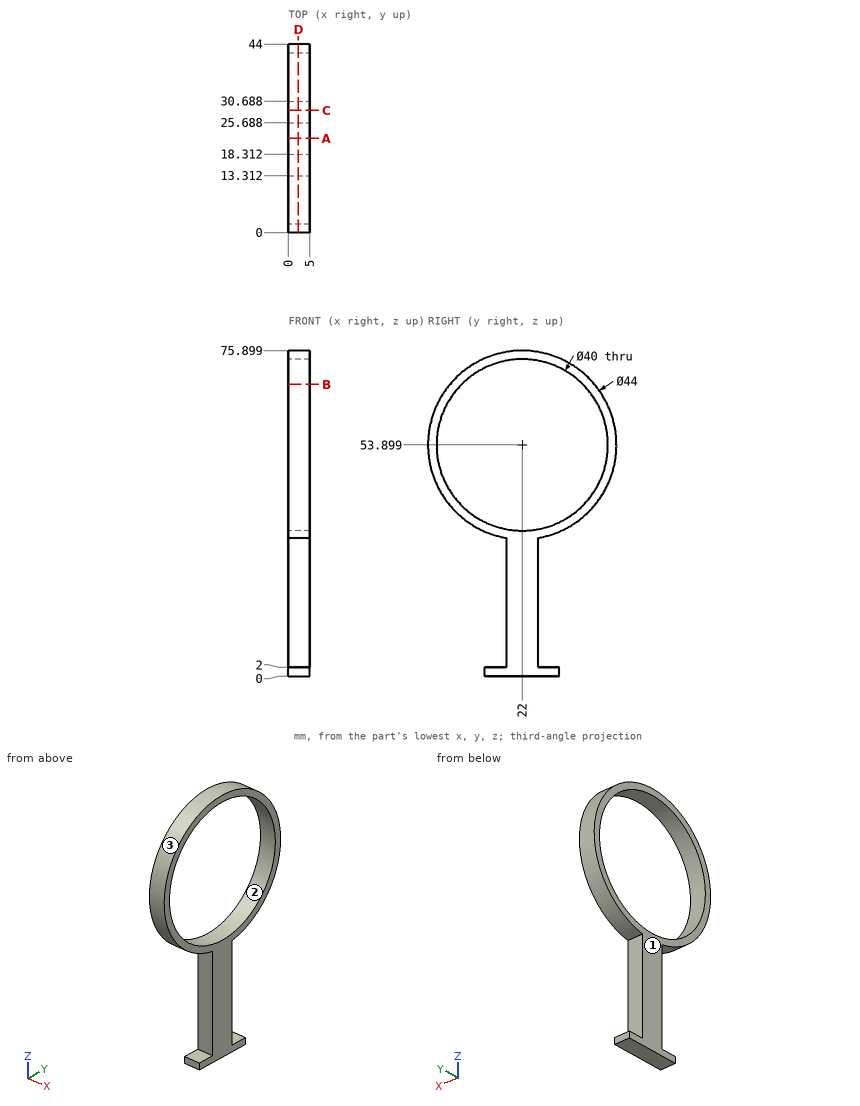
Part print with two shaded views. Sizes in mm from the minimum x, y, z corner. Give positions to 0.01 mm unless a question says otherwise; leave off trailing zeros. Order: outer loops, then holes, each group sorted by start corner. A loop starts at its lowest first (then second) coordinate and runs counter-clockwise, first axis right, second up.
1) Saw through at D-D, the plane x = 2.3. Write the cut outline in (y, z).
2) Mould opens along Y. For the marked faces 1, 2 and 3 say: +Y half, -Y half, draft (parallel to the pull), parting line (faces both ways), or undercut.
3) Wall check: probe 1 along Z at (x, y) = (2.05, 22); probe 2 along Z at (x, y) = (1.15, 20.5) (1 decimal); probe 3 along Y at (x, z) = (0.8, 15.5). Give the ranges that are in metal, low to high.
4) Pin check, flat tips, straight feed: pin 1 (12 mm diameter, centred on y = 31, z = 59.5, fed in from -X); pin 2 (2.5 mm diameter, centred on x = 2.5, z = 17.5, fed in from -Y); pin 3 (2 mm diameter, centred on x = 3, z = 0.5, fed in from +Y); pin 4 (1 mm diameter, centred on x = 3, z = 0.5, fed in from -Y). Stop position of each tip, or through.
5) Saw through at A-A, the plane y = 22. Write the cut outline in (x, z), then the cut area to 4 significant figures.
6) Saw through at C-C, the plane y = 28.5. Write the cut outline in (x, z), then the cut area to 3 significant figures.
7) Saw through at B-B, the plane z = 68. Write the cut outline in (x, y), then the cut area to 3 significant figures.
Computed:
1. outline: (13.31, 0) - (30.69, 0) - (30.69, 2) - (25.69, 2) - (25.69, 32.21) arc R22 ccw (long way) to (18.31, 32.21) - (18.31, 2) - (13.31, 2) - close; hole circle Ø40 at (22, 53.9)
2. face 1: draft
2. face 2: undercut
2. face 3: parting line
3. probe 1: z = 0 to 33.9, 73.9 to 75.9
3. probe 2: z = 0 to 34, 73.8 to 75.8
3. probe 3: y = 18.31 to 25.69
4. pin 1: passes through
4. pin 2: stops at y = 18.31
4. pin 3: stops at y = 30.69
4. pin 4: stops at y = 13.31
5. outline: (0, 0) - (5, 0) - (5, 33.9) - (0, 33.9) - close; (0, 73.9) - (5, 73.9) - (5, 75.9) - (0, 75.9) - close
5. area: 179.5 mm2
6. outline: (0, 0) - (5, 0) - (5, 2) - (0, 2) - close; (0, 32.88) - (5, 32.88) - (5, 34.98) - (0, 34.98) - close; (0, 72.81) - (5, 72.81) - (5, 74.92) - (0, 74.92) - close
6. area: 31.0 mm2
7. outline: (0, 5.11) - (5, 5.11) - (5, 7.82) - (0, 7.82) - close; (0, 36.18) - (5, 36.18) - (5, 38.89) - (0, 38.89) - close
7. area: 27.0 mm2
